For this review, use the dimensioned drawing (mm, ordinates from the lowest corner) and the shaded views. Coordinates: 2 decimals unless noted, no trailing zeros. Write each loop counter-clockwise with the first axis right and the second up, starting at its lowest first coordinate (ties: lowest second). Pieces come first, ordered by that corner, then holes. Notation, with made-up numbers: M -29.5,-13 L -20.5,-13 A20 cw -20.5,21 Z; hole C -12.75,82 d3. An arc over 180 degrees is marked long. One line per question, with ' | ' between items.
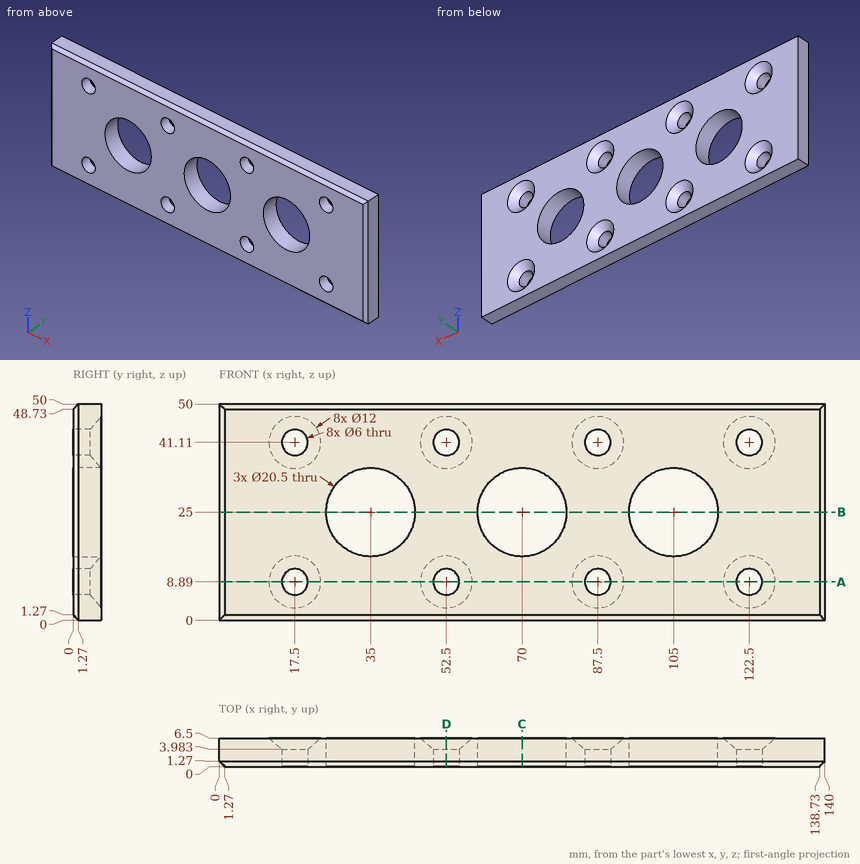
1) We need section C-C on x = 70. State the section outline as (y, z) points.
Responses:
outline: M 0,1.27 L 1.27,0 L 6.5,0 L 6.5,14.75 L 0,14.75 Z; M 0,35.25 L 6.5,35.25 L 6.5,50 L 1.27,50 L 0,48.73 Z
2) We need section A-A on z = 8.89. State how many separate pieces and enclosed holes the cut face has, then the cut area to 3 significant figures.
Responses:
separate pieces: 5 | enclosed holes: 0 | area: 722 mm^2
3) Insertion check: pin 1 Ø3.5 at (x, z) = (17.5, 8.89) entering from -Y; pin 2 Ø7 at (x, z) = (52.5, 8.89) entering from +Y; pin 3 Ø1 at (x, y) = (89.5, 1) entering from -Z; pin 4 Ø9.5 at (x, z) = (122.5, 8.89) entering from +Y. Each pin has a flat end and moves straight along its axis. Give the tip position at first contact, or say it passes through.
Responses:
pin 1: through | pin 2: y = 4.4 | pin 3: z = 0 | pin 4: y = 5.45
4) To check wall thickness, follow line 1 along Z through (x, y) = (52.5, 2.9); line 2 along X through (y, z) = (3.25, 25); line 3 along Z through (x, y) = (71.5, 5). State the ranges of each line that lie inside material, in increasing order. Write a range as [from, to].
Responses:
line 1: [0, 5.89], [11.89, 38.11], [44.11, 50] | line 2: [0, 24.75], [45.25, 59.75], [80.25, 94.75], [115.25, 140] | line 3: [0, 14.86], [35.14, 50]
5) We need section B-B on z = 25. State the section outline as (x, y) points, then the cut area to 3 significant figures.
Responses:
outline: M 0,1.27 L 1.27,0 L 24.75,0 L 24.75,6.5 L 0,6.5 Z; M 45.25,0 L 59.75,0 L 59.75,6.5 L 45.25,6.5 Z; M 80.25,0 L 94.75,0 L 94.75,6.5 L 80.25,6.5 Z; M 115.25,0 L 138.73,0 L 140,1.27 L 140,6.5 L 115.25,6.5 Z | area: 509 mm^2
6) We need section D-D on x = 52.5. State the section outline as (y, z) points.
Responses:
outline: M 0,1.27 L 1.27,0 L 6.5,0 L 6.5,2.89 L 3.98,5.89 L 0,5.89 Z; M 0,11.89 L 3.98,11.89 L 6.5,14.89 L 6.5,35.11 L 3.98,38.11 L 0,38.11 Z; M 0,44.11 L 3.98,44.11 L 6.5,47.11 L 6.5,50 L 1.27,50 L 0,48.73 Z
